For this review, take the finished solid that the model builds, in its own axes (mm). Face numbers are marked on the shaded views. A direction names the side the tool comes from. Coordinates: 2 decimals unless noted, no trailing zeros. Loops run counter-clockwise (first coordinate to the right, second up) from the corner with the lowest first, then second, coordinate; pieces in that order, holes last. Notation, with made-up numbers: (-12, 38) -> (39, 38) arc R18 cw to (39, 48) -> close; hole circle Ø2 at (75.25, -6). An arc over 180 degrees is marked (long way). Answer in a Markdown table with one row per item.
from build123d import *

# Parameters (mm, degrees)
F1_DEPTH = 82.55
F2_R     = 20.6375
F3_DEPTH = 12.701
F5_DEPTH = 25.401
F6_R     = 23.8125
F7_DEPTH = 25.401


with BuildPart() as f1:
    # F0 (on Front) → F1 (new body)
    with BuildSketch(Plane.XZ):
        Polygon((0, 101.6), (0, 0), (190.5, 0), (190.5, 12.7), (25.4, 12.7), (25.4, 101.6), align=None)
    extrude(amount=F1_DEPTH)

    # F2 (on face) → F3 (cut, through all)
    with BuildSketch(Plane.XY.offset(12.7)):
        with Locations((76.2, -41.275)):
            Circle(F2_R)
        with Locations((152.4, -41.275)):
            Circle(F2_R)
    extrude(amount=-F3_DEPTH, mode=Mode.SUBTRACT)

    # F4 (on face) → F5 (cut, through all)
    with BuildSketch(Plane.YZ.offset(25.4)):
        with BuildLine():
            Line((-82.55, 101.6), (-82.55, 69.85))
            ThreePointArc((-82.55, 69.85), (-41.275, 93.715476), (0, 69.85))
            Line((0, 69.85), (0, 101.6))
            Line((0, 101.6), (-82.55, 101.6))
        make_face()
    extrude(amount=-F5_DEPTH, mode=Mode.SUBTRACT)

    # F6 (on face) → F7 (cut, through all)
    with BuildSketch(Plane.YZ.offset(25.4)):
        with Locations((-41.275, 46.090476)):
            Circle(F6_R)
    extrude(amount=-F7_DEPTH, mode=Mode.SUBTRACT)


solid = f1.part
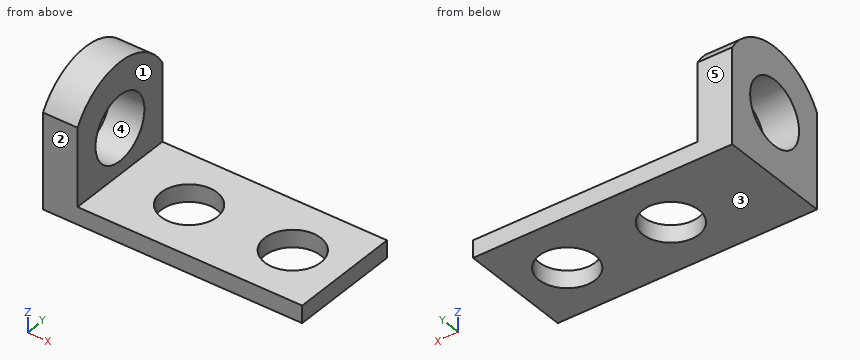
Item 1: Take a section at D-D, the plane x = 27.5. State the section outline as (y, z) points.
Worked answers:
| item | result |
|---|---|
| outline | (-82.55, 0) -> (0, 0) -> (0, 12.7) -> (-82.55, 12.7) -> close |
Item 2: Take a section at C-C, the plane y = -52. State the section outline as (x, z) points.
Worked answers:
| item | result |
|---|---|
| outline | (0, 0) -> (58.57, 0) -> (58.57, 12.7) -> (25.4, 12.7) -> (25.4, 24.83) -> (0, 24.83) -> close; (0, 67.35) -> (25.4, 67.35) -> (25.4, 92.49) -> (0, 92.49) -> close; (93.83, 0) -> (134.77, 0) -> (134.77, 12.7) -> (93.83, 12.7) -> close; (170.03, 0) -> (190.5, 0) -> (190.5, 12.7) -> (170.03, 12.7) -> close |
Item 3: For L1, parallel to Y at x = 152.4, z = 6.5; L2, parallel to X at y = -40, z = 10; L3, parallel to Z at x = 22, y = -42, list the stretches that pass through material, from the lowest coordinate up.
Worked answers:
| item | result |
|---|---|
| L1 | -82.55 to -61.91, -20.64 to 0 |
| L2 | 0 to 55.6, 96.8 to 131.8, 173 to 190.5 |
| L3 | 0 to 22.29, 69.89 to 93.71 |
Item 4: Insertion check: pin 1 (10 mm diameter, centred on x = 91, y = -36, fed in from +Z); pin 2 (12 mm diameter, centred on y = -15.5, z = 20.5, fed in from +X). Each pin has a flat end and moves straight along its axis. Give the tip position at first contact, or say it passes through.
Worked answers:
| item | result |
|---|---|
| pin 1 | z = 12.7 |
| pin 2 | x = 25.4 |
Item 5: Take a section at A-A, the plane x = 159.5. State the section outline as (y, z) points, and give its area (3 significant figures).
Worked answers:
| item | result |
|---|---|
| outline | (-82.55, 0) -> (-60.65, 0) -> (-60.65, 12.7) -> (-82.55, 12.7) -> close; (-21.9, 0) -> (0, 0) -> (0, 12.7) -> (-21.9, 12.7) -> close |
| area | 556 mm² |
Item 6: The part is to be moulded in two halves that separate along Y. For the marked faces 3, 4 and 5, say which applies: +Y half, -Y half, draft (parallel to the pull), parting line (faces both ways), or undercut.
Worked answers:
| item | result |
|---|---|
| face 3 | draft |
| face 4 | undercut |
| face 5 | +Y half |
Item 7: For the marked faces 1 and 2, list the 3-axis set-ups (+Z, -Z, +X, -X, +Y, -Y) from which the entire face can be reached by the end or side of a thin tool; tool diameter is ignored.
Worked answers:
| item | result |
|---|---|
| face 1 | +Z, +X, +Y, -Y |
| face 2 | +Z, -Z, +X, -X, -Y |
Item 8: Take a section at B-B, the plane z = 64.5. State the section outline as (x, y) points.
Worked answers:
| item | result |
|---|---|
| outline | (0, -82.55) -> (25.4, -82.55) -> (25.4, -56.38) -> (0, -56.38) -> close; (0, -26.17) -> (25.4, -26.17) -> (25.4, 0) -> (0, 0) -> close |
